The listing builds one solid part. Answer for the finished solid, in the listing's coordinates (mm). A direction names the side the tool comes from. Coordinates: 2 decimals unless noted, no trailing zeros. Order: outer loops, then holes, each group sorted by start corner. A loop starts at its lowest first (then second) coordinate and runs counter-clockwise, first axis right, second up. Notation, with made-up numbers: (32.25, 62.5) -> (51.25, 62.5) arc R13 cw to (51.25, 66.5) -> close; hole circle Ø6 at (84.25, 75). An arc over 180 degrees is marked (long way). Return JSON: item names as keys, results as strings.
```python
from build123d import *

# Parameters (mm, degrees)
F1_DEPTH = 1


with BuildPart() as f1:
    # F0 (on Top) → F1 (new body)
    with BuildSketch(Plane.XY):
        with BuildLine():
            Line((-22.392857, 32), (-20.068879, -33.071383))
            ThreePointArc((-20.068879, -33.071383), (-19.4589, -34.43923), (-18.070153, -35))
            Line((-18.070153, -35), (18.070153, -35))
            ThreePointArc((18.070153, -35), (19.4589, -34.43923), (20.068879, -33.071383))
            Line((20.068879, -33.071383), (22.392857, 32))
            Line((22.392857, 32), (22.426022, 32.928617))
            ThreePointArc((22.426022, 32.928617), (21.866526, 34.388747), (20.427296, 35))
            Line((20.427296, 35), (7, 35))
            ThreePointArc((7, 35), (5.585786, 35.585786), (5, 37))
            Line((5, 37), (5, 55))
            Line((5, 55), (-5, 55))
            Line((-5, 55), (-5, 37))
            ThreePointArc((-5, 37), (-5.585786, 35.585786), (-7, 35))
            Line((-7, 35), (-20.427296, 35))
            ThreePointArc((-20.427296, 35), (-21.866526, 34.388747), (-22.426022, 32.928617))
            Line((-22.426022, 32.928617), (-22.392857, 32))
        make_face()
        with BuildLine():
            Line((-16.32887, -28.869881), (16.206912, -24.007376))
            ThreePointArc((16.206912, -24.007376), (17.020899, -24.250598), (17.354084, -25.032083))
            Line((17.354084, -25.032083), (17.174109, -30.071383))
            ThreePointArc((17.174109, -30.071383), (16.56413, -31.43923), (15.175384, -32))
            Line((15.175384, -32), (-15.175384, -32))
            ThreePointArc((-15.175384, -32), (-16.56413, -31.43923), (-17.174109, -30.071383))
            Line((-17.174109, -30.071383), (-17.180423, -29.894589))
            ThreePointArc((-17.180423, -29.894589), (-16.950156, -29.219763), (-16.32887, -28.869881))
        make_face(mode=Mode.SUBTRACT)
        with BuildLine():
            Line((-16.688062, -18.812502), (16.569959, -13.842057))
            ThreePointArc((16.569959, -13.842057), (17.383946, -14.085279), (17.717131, -14.866764))
            Line((17.717131, -14.866764), (17.571913, -18.932892))
            ThreePointArc((17.571913, -18.932892), (17.318343, -19.563378), (16.720359, -19.886216))
            Line((16.720359, -19.886216), (-16.248766, -24.813485))
            ThreePointArc((-16.248766, -24.813485), (-17.03571, -24.593564), (-17.395939, -23.860161))
            Line((-17.395939, -23.860161), (-17.539616, -19.837209))
            ThreePointArc((-17.539616, -19.837209), (-17.309348, -19.162383), (-16.688062, -18.812502))
        make_face(mode=Mode.SUBTRACT)
        with BuildLine():
            Line((-17.047254, -8.755122), (16.933006, -3.676738))
            ThreePointArc((16.933006, -3.676738), (17.746993, -3.91996), (18.080179, -4.701445))
            Line((18.080179, -4.701445), (17.93496, -8.767573))
            ThreePointArc((17.93496, -8.767573), (17.68139, -9.398059), (17.083406, -9.720897))
            Line((17.083406, -9.720897), (-16.607959, -14.756106))
            ThreePointArc((-16.607959, -14.756106), (-17.394902, -14.536185), (-17.755131, -13.802781))
            Line((-17.755131, -13.802781), (-17.898808, -9.779829))
            ThreePointArc((-17.898808, -9.779829), (-17.66854, -9.105003), (-17.047254, -8.755122))
        make_face(mode=Mode.SUBTRACT)
        with BuildLine():
            Line((-17.406446, 1.302258), (17.296053, 6.488581))
            ThreePointArc((17.296053, 6.488581), (18.11004, 6.245359), (18.443226, 5.463874))
            Line((18.443226, 5.463874), (18.298007, 1.397746))
            ThreePointArc((18.298007, 1.397746), (18.044437, 0.76726), (17.446453, 0.444422))
            Line((17.446453, 0.444422), (-16.967151, -4.698726))
            ThreePointArc((-16.967151, -4.698726), (-17.754094, -4.478805), (-18.114323, -3.745402))
            Line((-18.114323, -3.745402), (-18.258, 0.27755))
            ThreePointArc((-18.258, 0.27755), (-18.027732, 0.952376), (-17.406446, 1.302258))
        make_face(mode=Mode.SUBTRACT)
        with BuildLine():
            ThreePointArc((12.16906, 32), (13.16631, 31.074108), (12.31687, 30.010984))
            Line((12.31687, 30.010984), (-16.937512, 25.638888))
            ThreePointArc((-16.937512, 25.638888), (-18.511399, 26.078729), (-19.231856, 27.545536))
            Line((-19.231856, 27.545536), (-19.316967, 29.928617))
            ThreePointArc((-19.316967, 29.928617), (-18.757471, 31.388747), (-17.318241, 32))
            Line((-17.318241, 32), (12.16906, 32))
        make_face(mode=Mode.SUBTRACT)
        with BuildLine():
            Line((-17.765639, 11.359637), (17.659101, 16.6539))
            ThreePointArc((17.659101, 16.6539), (18.473087, 16.410678), (18.806273, 15.629193))
            Line((18.806273, 15.629193), (18.661054, 11.563065))
            ThreePointArc((18.661054, 11.563065), (18.407485, 10.932579), (17.809501, 10.609741))
            Line((17.809501, 10.609741), (-17.326343, 5.358654))
            ThreePointArc((-17.326343, 5.358654), (-18.113287, 5.578575), (-18.473515, 6.311978))
            Line((-18.473515, 6.311978), (-18.617192, 10.33493))
            ThreePointArc((-18.617192, 10.33493), (-18.386924, 11.009756), (-17.765639, 11.359637))
        make_face(mode=Mode.SUBTRACT)
        with BuildLine():
            Line((-18.124831, 21.417017), (18.022148, 26.819219))
            ThreePointArc((18.022148, 26.819219), (18.836134, 26.575997), (19.16932, 25.794512))
            Line((19.16932, 25.794512), (19.024101, 21.728384))
            ThreePointArc((19.024101, 21.728384), (18.770532, 21.097898), (18.172548, 20.77506))
            Line((18.172548, 20.77506), (-17.685535, 15.416033))
            ThreePointArc((-17.685535, 15.416033), (-18.472479, 15.635954), (-18.832707, 16.369358))
            Line((-18.832707, 16.369358), (-18.976384, 20.39231))
            ThreePointArc((-18.976384, 20.39231), (-18.746116, 21.067135), (-18.124831, 21.417017))
        make_face(mode=Mode.SUBTRACT)
    extrude(amount=F1_DEPTH)


solid = f1.part
```
Item 1: Find the intervals of material crossed by probe 1 along X at (y, z) = (46, 0.3); probe 2 along X at (y, z) = (-29.5, 0.6); probe 3 along X at (y, z) = (11, 0.8), in increasing order.
Answer list:
{"probe 1": "-5 to 5", "probe 2": "-20.2 to -17.11, 17.19 to 20.2", "probe 3": "-21.64 to -18.39, 18.46 to 21.64"}
Item 2: Which of the six approach directions +Z, -Z, +X, -X, +Y, -Y give full straight-line access (tool end or side, diameter ignored) to faces 4 (the cylindrical face through (-19.5, -34.4, 0.5)), 5 (the cylindrical face through (16.58, -31.424, 0.493))?
Answer list:
{"face 4": "+Z, -Z, -X, -Y", "face 5": "+Z, -Z"}
Item 3: Flat-ended cylindrical pins translate along their axes: pin 1 (0.5 mm diameter, centred on y = 45, z = 0.5, fed in from +X); pin 2 (0.5 mm diameter, centred on x = -7, z = 0.5, fed in from +Y). Find the tip coordinate at first contact, or state that the pin passes through.
Answer list:
{"pin 1": "x = 5", "pin 2": "y = 35.02"}
Item 4: Determine the mould class of faces 1 (the flat face through (-0.289, -26.473, 0.493)), 2 (the cylindrical face through (19.443, -34.454, 0.493)), 3 (the flat face through (-2, 7, 0)) for opening direction Y: pulls with the +Y half, pulls with the -Y half, needs draft (parallel to the pull), parting line crosses it, or undercut.
Answer list:
{"face 1": "undercut", "face 2": "pulls with the -Y half", "face 3": "needs draft"}
Item 5: The part is cut by section B-B on y = -21.5. Determine the outline of the cut face in (x, z).
Answer list:
{"outline": "(-20.48, 0) -> (-17.48, 0) -> (-17.48, 1) -> (-20.48, 1) -> close; (5.92, 0) -> (20.48, 0) -> (20.48, 1) -> (5.92, 1) -> close"}
Item 6: The part is cut by section A-A on x = 0. Count the separate pieces of the cut face and the enclosed holes in it, plus the area to 3 significant figures.
Answer list:
{"separate pieces": "8", "enclosed holes": "0", "area": "50.3 mm2"}
